Input: part model. Units: mm. Frame: model coordinates. Face numbers are marked on the shaded views. A direction names the side the tool comes from. Coordinates: 2 decimals unless noted, no trailing zeros. Write each loop counter-clockwise with the first axis right and the second up, starting at its lowest first coordinate (ties: lowest second). Pieces come first, ordered by that corner, then holes. Notation, with made-up numbers: (27, 74) -> (52, 74) arc R21 ccw to (52, 101) -> close; hole circle Ø7 at (81, 13). An arc over 180 degrees is marked (long way). Use one line per item in the form item = value. Start each with the question number.
(1) Cut plane A-A on x = 8. Return the cut outline in (y, z), plus the area to 3 significant figures.
(2) First-contact query: pin 1 (2 mm diameter, centred on y = -39, z = 31, fed in from -X); pin 2 (1 mm diameter, centred on x = -13, y = -21, fed in from +Z); pin 3 (2.5 mm diameter, centred on x = -13, y = -13.5, fed in from -Z). Flat tips, straight axial feed; report the tip coordinate or a pass-through.
(3) Cut plane C-C on y = -33.5. Return the cut outline in (x, z).
(4) Cut plane B-B on z = 37. Return the cut outline in (x, y).
(5) Ray query, line 1 along Y through (x, z) = (31, 41); line 2 along Z through (x, y) = (4, 4); line 3 along X through (y, z) = (-1.5, 39.5). Return the intervals inside material, ascending.
(6) Cut plane D-D on z = 4. Return the cut outline in (x, y), plus the area to 3 significant figures.
(7) Set-up query: the marked faces 1, 2, 3, 4 and 5. Return all of +Z, -Z, +X, -X, +Y, -Y with unobstructed straight access to the full face (end or side cutting, diameter ignored); none if empty.
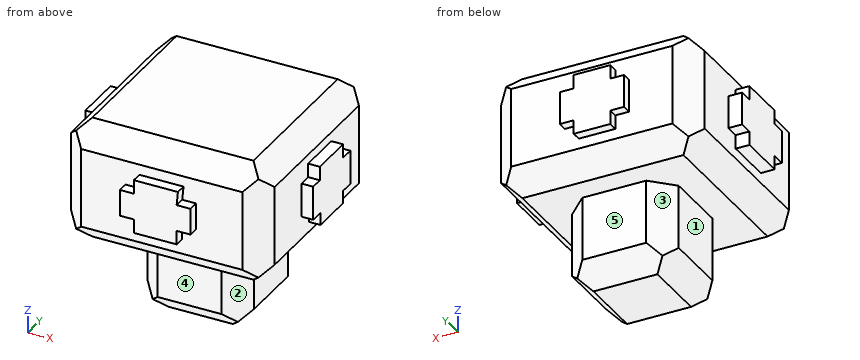
```python
from build123d import *

# Parameters (mm, degrees)
F0_W      = 25.41670762
F0_H      = 25.4167113453
F1_DEPTH  = 26.416
F2_SIZE   = 5.08
F3_SIZE   = 5.08
F4_SIZE   = 5.08
F5_SIZE   = 5.08
F6_SIZE   = 5.08
F7_SIZE   = 5.08
F8_SIZE   = 5.08
F9_SIZE   = 5.08
F10_SIZE  = 5.08
F11_SIZE  = 5.08
F12_SIZE  = 5.08
F13_SIZE  = 5.08
F14_W     = 48.5844528303
F14_H     = 48.3157048002
F15_DEPTH = 6.096
F16_DEPTH = 23.114
F17_SIZE  = 5.08
F18_SIZE  = 5.08
F19_SIZE  = 5.08
F20_SIZE  = 5.08
F21_SIZE  = 5.08
F22_SIZE  = 5.08
F23_SIZE  = 5.08
F24_SIZE  = 5.08
F25_SIZE  = 5.08
F26_SIZE  = 5.08
F27_SIZE  = 5.08
F29_DEPTH = 2.54
F31_DEPTH = 2.286
F33_DEPTH = 2.794
F35_DEPTH = 3.302


with BuildPart() as f1:
    # F0 (on Top) → F1 (new body)
    with BuildSketch(Plane.XY):
        with Locations((12.70835381, -12.7083556727)):
            Rectangle(F0_W, F0_H)
    extrude(amount=F1_DEPTH)

    # F2
    f2_edges = [f1.edges().sort_by_distance(p)[0] for p in [
        (12.708354, -25.416711, 0),
    ]]
    chamfer(f2_edges, length=F2_SIZE)

    # F3
    f3_edges = [f1.edges().sort_by_distance(p)[0] for p in [
        (12.708354, 0, 0),
    ]]
    chamfer(f3_edges, length=F3_SIZE)

    # F4
    f4_edges = [f1.edges().sort_by_distance(p)[0] for p in [
        (12.708354, 0, 26.416),
    ]]
    chamfer(f4_edges, length=F4_SIZE)

    # F5
    f5_edges = [f1.edges().sort_by_distance(p)[0] for p in [
        (12.708354, -25.416711, 26.416),
    ]]
    chamfer(f5_edges, length=F5_SIZE)

    # F6
    f6_edges = [f1.edges().sort_by_distance(p)[0] for p in [
        (25.416708, 0, 13.208),
    ]]
    chamfer(f6_edges, length=F6_SIZE)

    # F7
    f7_edges = [f1.edges().sort_by_distance(p)[0] for p in [
        (0, 0, 13.208),
    ]]
    chamfer(f7_edges, length=F7_SIZE)

    # F8
    f8_edges = [f1.edges().sort_by_distance(p)[0] for p in [
        (0, -25.416711, 13.208),
    ]]
    chamfer(f8_edges, length=F8_SIZE)

    # F9
    f9_edges = [f1.edges().sort_by_distance(p)[0] for p in [
        (25.416708, -25.416711, 13.208),
    ]]
    chamfer(f9_edges, length=F9_SIZE)

    # F10
    f10_edges = [f1.edges().sort_by_distance(p)[0] for p in [
        (25.416708, -12.708356, 0),
    ]]
    chamfer(f10_edges, length=F10_SIZE)

    # F11
    f11_edges = [f1.edges().sort_by_distance(p)[0] for p in [
        (25.416708, -12.708356, 26.416),
    ]]
    chamfer(f11_edges, length=F11_SIZE)

    # F12
    f12_edges = [f1.edges().sort_by_distance(p)[0] for p in [
        (0, -12.708356, 0),
    ]]
    chamfer(f12_edges, length=F12_SIZE)

    # F13
    f13_edges = [f1.edges().sort_by_distance(p)[0] for p in [
        (0, -12.708356, 26.416),
    ]]
    chamfer(f13_edges, length=F13_SIZE)

    # F14 (on face) → F15 (join)
    with BuildSketch(Plane.XY.offset(26.416)):
        with Locations((12.3993125744, -13.3544201963)):
            Rectangle(F14_W, F14_H)
    extrude(amount=-F15_DEPTH)

    # F16 (add): a face of the model
    f16_faces = [f1.faces().sort_by_distance(p)[0] for p in [
        (12.3993125744, -13.3544201963, 26.416),
    ]]
    extrude(f16_faces, amount=F16_DEPTH)

    # F17
    f17_edges = [f1.edges().sort_by_distance(p)[0] for p in [
        (-11.892914, -37.512273, 34.925),
    ]]
    chamfer(f17_edges, length=F17_SIZE)

    # F18
    f18_edges = [f1.edges().sort_by_distance(p)[0] for p in [
        (14.939313, -37.512273, 49.53),
        (14.939313, -37.512273, 20.32),
    ]]
    chamfer(f18_edges, length=F18_SIZE)

    # F19
    f19_edges = [f1.edges().sort_by_distance(p)[0] for p in [
        (36.691539, -37.512273, 34.925),
    ]]
    chamfer(f19_edges, length=F19_SIZE)

    # F20
    f20_edges = [f1.edges().sort_by_distance(p)[0] for p in [
        (36.691539, -10.81442, 49.53),
    ]]
    chamfer(f20_edges, length=F20_SIZE)

    # F21
    f21_edges = [f1.edges().sort_by_distance(p)[0] for p in [
        (36.691539, -10.81442, 20.32),
    ]]
    chamfer(f21_edges, length=F21_SIZE)

    # F22
    f22_edges = [f1.edges().sort_by_distance(p)[0] for p in [
        (36.691539, 10.803432, 34.925),
    ]]
    chamfer(f22_edges, length=F22_SIZE)

    # F23
    f23_edges = [f1.edges().sort_by_distance(p)[0] for p in [
        (9.859313, 10.803432, 49.53),
    ]]
    chamfer(f23_edges, length=F23_SIZE)

    # F24
    f24_edges = [f1.edges().sort_by_distance(p)[0] for p in [
        (9.859313, 10.803432, 20.32),
    ]]
    chamfer(f24_edges, length=F24_SIZE)

    # F25
    f25_edges = [f1.edges().sort_by_distance(p)[0] for p in [
        (-11.892914, 10.803432, 34.925),
    ]]
    chamfer(f25_edges, length=F25_SIZE)

    # F26
    f26_edges = [f1.edges().sort_by_distance(p)[0] for p in [
        (-11.892914, -13.35442, 49.53),
    ]]
    chamfer(f26_edges, length=F26_SIZE)

    # F27
    f27_edges = [f1.edges().sort_by_distance(p)[0] for p in [
        (-11.892914, -13.35442, 20.32),
    ]]
    chamfer(f27_edges, length=F27_SIZE)

    # F28 (on face) → F29 (join)
    with BuildSketch(Plane.XZ.offset(37.5122725964)):
        Polygon((17.5961852074, 41.9601351023), (7.0685530081, 41.9601351023), (7.0685530081, 38.6514477432), (3.7598696072, 38.6514477432), (3.7598696072, 32.3348678648), (7.0685530081, 32.3348678648), (7.0685530081, 29.026184231), (17.2953959554, 29.026184231), (17.2953959554, 32.3348678648), (20.6040795892, 32.3348678648), (20.6040795892, 38.6514477432), (17.2953959554, 38.6514477432), align=None)
    extrude(amount=F29_DEPTH)

    # F30 (on face) → F31 (join)
    with BuildSketch(Plane(origin=(0, 10.8034322038, 0), x_dir=(-1, 0, 0), z_dir=(0, 1, 0))):
        Polygon((-6.7677642219, 38.9522351325), (-6.7677642219, 42.2609224916), (-15.4906576499, 42.2609224916), (-15.4906576499, 38.9522351325), (-18.7993440777, 38.9522351325), (-18.7993440777, 31.1317108572), (-15.4906576499, 31.1317108572), (-15.4906576499, 27.8230272233), (-6.7677642219, 27.8230272233), (-6.7677642219, 31.1317108572), (-3.4590810537, 31.1317108572), (-3.4590810537, 38.9522351325), align=None)
    extrude(amount=F31_DEPTH)

    # F32 (on face) → F33 (join)
    with BuildSketch(Plane.YZ.offset(36.6915389895)):
        Polygon((-6.7677642219, 38.9522351325), (-6.7677642219, 42.2609224916), (-17.2953940928, 42.2609224916), (-17.2953940928, 38.9522351325), (-20.3032903373, 38.9522351325), (-20.3032903373, 30.8309197426), (-16.9946048409, 30.8309197426), (-16.9946048409, 27.8230272233), (-6.7677642219, 27.8230272233), (-6.7677642219, 30.8309197426), (-3.4590810537, 30.8309197426), (-3.4590810537, 38.9522351325), align=None)
    extrude(amount=F33_DEPTH)

    # F34 (on face) → F35 (join)
    with BuildSketch(Plane(origin=(-11.8929138407, 0, 0), x_dir=(0, -1, 0), z_dir=(-1, 0, 0))):
        Polygon((19.7017118335, 42.2609224916), (8.2717109472, 42.2609224916), (8.2717109472, 38.9522351325), (4.9630273134, 38.9522351325), (4.9630273134, 31.1317108572), (8.2717109472, 31.1317108572), (8.2717109472, 27.8230272233), (19.7017118335, 27.8230272233), (19.7017118335, 31.1317108572), (23.0103954673, 31.1317108572), (23.0103954673, 38.9522351325), (19.7017118335, 38.9522351325), align=None)
    extrude(amount=F35_DEPTH)


solid = f1.part
```
Values:
q1.outline = (-40.05, 29.03) -> (-37.51, 29.03) -> (-37.51, 25.4) -> (-32.43, 20.32) -> (-25.42, 20.32) -> (-25.42, 5.08) -> (-20.34, 0) -> (-5.08, 0) -> (0, 5.08) -> (0, 20.32) -> (5.72, 20.32) -> (10.8, 25.4) -> (10.8, 27.82) -> (13.09, 27.82) -> (13.09, 42.26) -> (10.8, 42.26) -> (10.8, 44.45) -> (5.72, 49.53) -> (-32.43, 49.53) -> (-37.51, 44.45) -> (-37.51, 41.96) -> (-40.05, 41.96) -> close
q1.area = 1,920 mm2
q2.pin_1 = 7.07
q2.pin_2 = 38.95
q2.pin_3 = 25.26
q3.outline = (-10.83, 24.33) -> (-7.88, 21.39) -> (32.68, 21.39) -> (35.62, 24.33) -> (35.62, 45.52) -> (32.68, 48.46) -> (-7.88, 48.46) -> (-10.83, 45.52) -> close
q4.outline = (-15.19, -23.01) -> (-11.89, -23.01) -> (-11.89, -32.43) -> (-6.81, -37.51) -> (3.76, -37.51) -> (3.76, -40.05) -> (20.6, -40.05) -> (20.6, -37.51) -> (31.61, -37.51) -> (36.69, -32.43) -> (36.69, -20.3) -> (39.49, -20.3) -> (39.49, -3.46) -> (36.69, -3.46) -> (36.69, 5.72) -> (31.61, 10.8) -> (18.8, 10.8) -> (18.8, 13.09) -> (3.46, 13.09) -> (3.46, 10.8) -> (-6.81, 10.8) -> (-11.89, 5.72) -> (-11.89, -4.96) -> (-15.19, -4.96) -> close
q5.line_1 = -37.51 to 10.8
q5.line_2 = 20.32 to 49.53
q5.line_3 = -11.89 to 36.69
q6.outline = (1.08, -21.42) -> (4, -24.34) -> (21.42, -24.34) -> (24.34, -21.42) -> (24.34, -4) -> (21.42, -1.08) -> (4, -1.08) -> (1.08, -4) -> close
q6.area = 524 mm2
q7.face_1 = -Z, -X, +Y, -Y
q7.face_2 = -Z, +X, -Y
q7.face_3 = -Z, -X, +Y
q7.face_4 = -Z, +X, -X, -Y
q7.face_5 = -Z, +X, -X, +Y
